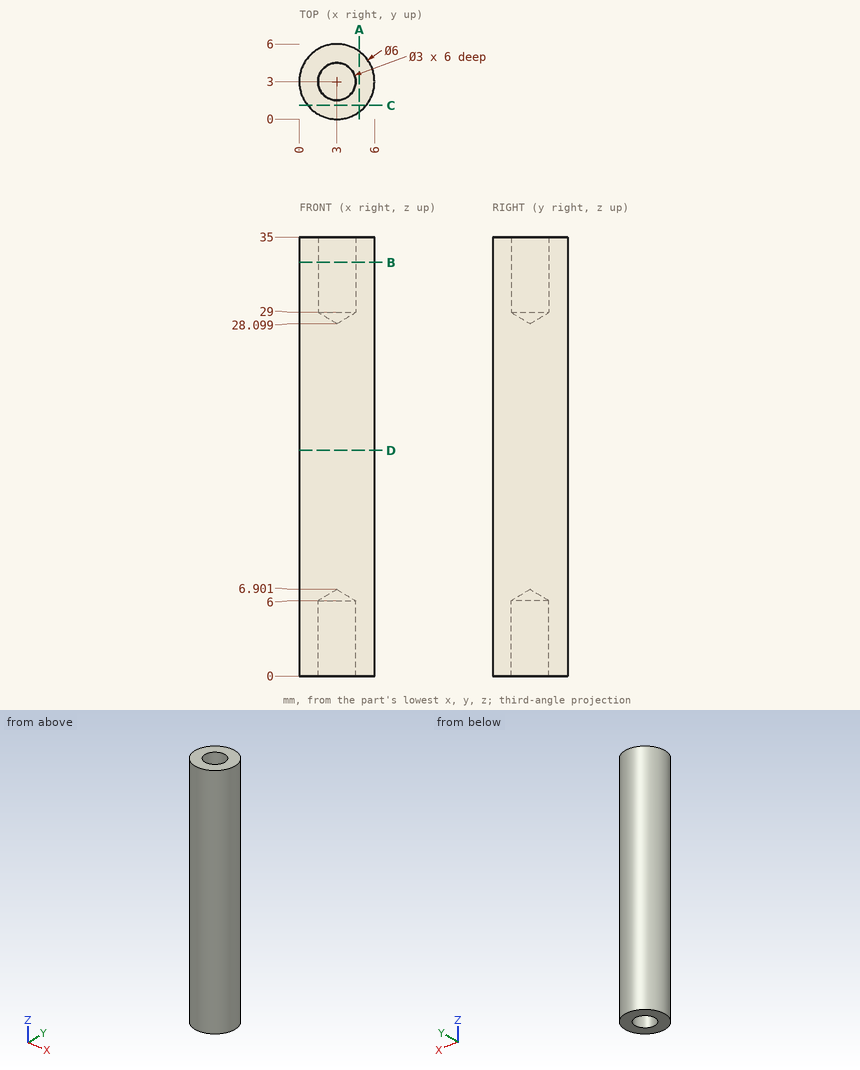
The drawing under review shows one solid part. Ordinate dimensions are in mm from its lowest x, y, z. Coordinates: 2 decimals unless noted, no trailing zeros. Loops run counter-clockwise (first coordinate to the right, second up) from the corner with the lowest first, then second, coordinate; pieces in that order, holes last. Notation, with made-up numbers: (54, -21.75) -> (95, -21.75) arc R21 ccw to (95, -9.75) -> close; hole circle Ø2 at (8.25, 89.5). An arc over 180 degrees is marked (long way). Answer as a JSON object with one key per item and string values.
Q1. Take a section at C-C on y = 1.1. Give the boundary of the cut face in (x, z).
Answer block:
{"outline": "(0.68, 0) -> (5.32, 0) -> (5.32, 35) -> (0.68, 35) -> close"}
Q2. Take a section at A-A on x = 4.8. Give the boundary of the cut face in (y, z), plus the area to 3 significant figures.
Answer block:
{"outline": "(0.6, 0) -> (5.4, 0) -> (5.4, 35) -> (0.6, 35) -> close", "area": "168 mm^2"}
Q3. Take a section at B-B on z = 33. Give the boundary of the cut face in (x, y), plus the area to 3 significant figures.
Answer block:
{"outline": "circle Ø6 at (3, 3); hole circle Ø3 at (3, 3)", "area": "21.2 mm^2"}
Q4. To check wall thickness, follow L1, parallel to Y at x = 3, z = 1.7; L2, parallel to X at y = 2.9, z = 10. State the ranges of each line that lie inside material, in increasing order.
Answer block:
{"L1": "y = 0 to 1.5, 4.5 to 6", "L2": "x = 0 to 6"}
Q5. Take a section at D-D on z = 18. Give the boundary of the cut face in (x, y), plus the area to 3 significant figures.
Answer block:
{"outline": "circle Ø6 at (3, 3)", "area": "28.3 mm^2"}
Q6. Clearance check with flat-ended pins moving along their axes: pin 1 Ø1 at (y, z) = (4, 6.5) entering from -X; pin 2 Ø1 at (x, z) = (1.5, 16.5) entering from +Y; pin 3 Ø1.8 at (x, y) = (3, 3) entering from +Z. State where each tip first meets the part, or that it passes through.
Answer block:
{"pin 1": "stops at x = 0.04", "pin 2": "stops at y = 5.83", "pin 3": "stops at z = 28.64"}
